Solid Edge part; units mm, degrees
sketch "Sketch1" plane through (0, 0, 0) normal (0, 0, 1) x (1, 0, 0)
  line L0 (524.9437, -191.5504) -> (1813.8262, -660.6653)
  line L1 (0.4572, -1930.4) -> (0.4572, -558.7998)
  arc A0 (1813.8262, -660.6653) -> (0.4572, -1930.4) centre (-0.0001, 0) cw
  arc A1 (524.9437, -191.5504) -> (0.4572, -558.7998) centre (0, 0) cw
  circle A2 centre (713.8732, -1019.5166) radius 647.7
extrude "Protrusion1" add sketch "Sketch1" along normal blind 6.35
Here's how the part is built. I have some questions about the finished solid (model axes, mm). Coordinates: 2 decimals unless noted, no trailing zeros. Order: outer loops, then holes, each group sorted by start corner. A loop starts at its lowest first (then second) coordinate and runs counter-clockwise, first axis right, second up. Notation, with made-up numbers: (44.25, -32) -> (68.25, -32) arc R20 cw to (68.25, -23) -> close; hole circle Ø1 at (49, 20.5). An arc over 180 degrees is marked (long way). Answer in a Markdown table with one row per item.
(1) Please list where these lines run through material, in increasing order: probe 1 along Y at (x, z) = (612, 1.75); probe 2 along X at (y, z) = (-1522.5, 1.5); probe 3 along X at (y, z) = (-1197, 1).
Answer key:
| item | result |
|---|---|
| probe 1 | -1830.82 to -1659.15, -379.88 to -223.24 |
| probe 2 | 0.46 to 305.8, 1121.95 to 1186.78 |
| probe 3 | 0.46 to 90.96, 1336.78 to 1514.48 |
(2) I want a section at D-D on x = 1682.5. List the corners of the cut face in (y, z) for me, then the cut area to 3 significant figures.
Answer key:
| item | result |
|---|---|
| outline | (-946.38, 0) -> (-612.87, 0) -> (-612.87, 6.35) -> (-946.38, 6.35) -> close |
| area | 2,120 mm^2 |
(3) Thinking about a two-plate mould opening in Y: for faces 1 (the face through (1160.363, -422.824, 3.131)), 2 (the face through (1120.709, -1571.768, 3.131)), 3 (the face through (1062.07, -1565.66, 3.13)), which applies, +Y half, -Y half, draft (parallel to the pull), parting line (faces both ways), or undercut?
Answer key:
| item | result |
|---|---|
| face 1 | +Y half |
| face 2 | -Y half |
| face 3 | undercut |
(4) I want a section at A-A on x = 497.5. List the corners of the cut face in (y, z) for me, then the cut area to 3 significant figures.
Answer key:
| item | result |
|---|---|
| outline | (-1865.19, 0) -> (-1630.01, 0) -> (-1630.01, 6.35) -> (-1865.19, 6.35) -> close; (-409.03, 0) -> (-254.46, 0) -> (-254.46, 6.35) -> (-409.03, 6.35) -> close |
| area | 2,470 mm^2 |
(5) I want a section at C-C on z = 3. List the corners of the cut face in (x, y) for me.
Answer key:
| item | result |
|---|---|
| outline | (0.46, -1930.4) arc R1930.4 ccw to (1813.83, -660.67) -> (524.94, -191.55) arc R558.8 cw to (0.46, -558.8) -> close; hole circle Ø1295.4 at (713.87, -1019.52) |
(6) I want a section at B-B on y = -475. List the corners of the cut face in (x, z) for me, then the cut area to 3 significant figures.
Answer key:
| item | result |
|---|---|
| outline | (294.33, 0) -> (363.14, 0) -> (363.14, 6.35) -> (294.33, 6.35) -> close; (1064.61, 0) -> (1303.72, 0) -> (1303.72, 6.35) -> (1064.61, 6.35) -> close |
| area | 1,960 mm^2 |
